Here's how the part is built. I have some questions about the finished solid (model axes, mm). Face numbers are marked on the shaded views. Coordinates: 2 decimals unless noted, no trailing zeros. Write each loop counter-clockwise with the first axis right and the second up, starting at its lowest first coordinate (ties: lowest second). Pieces come first, ordered by that corner, then holes. Notation, with made-up numbers: M 66.5,-37.75 L 85.5,-37.75 A32 ccw 85.5,-4.75 Z; hole C 31,9.5 d6. An arc over 180 degrees is marked long. Use a Markdown table: item, result.
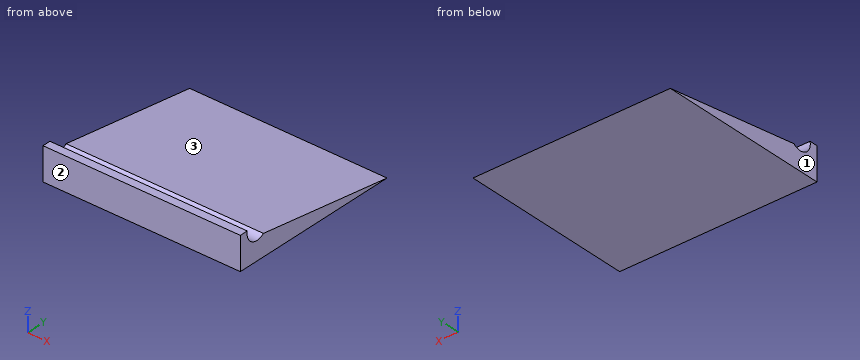
```python
from build123d import *

# Parameters (mm, degrees)
F1_DEPTH = 152.4


with BuildPart() as f1:
    # F0 (on Right) → F1 (new body)
    with BuildSketch(Plane.YZ):
        with BuildLine():
            Line((-92.604421, 0.601124), (-90.45029, 0.601124))
            Line((-90.45029, 0.601124), (41.62971, 0.601124))
            Line((41.62971, 0.601124), (-71.477041, 17.073922))
            ThreePointArc((-71.477041, 17.073922), (-82.034408, 16.292348), (-86.254421, 26.001124))
            Line((-86.254421, 26.001124), (-92.604421, 26.001124))
            Line((-92.604421, 26.001124), (-92.604421, 0.601124))
        make_face()
    extrude(amount=-F1_DEPTH)


solid = f1.part
```
1. Suppose I cut it at B-B on y = -32.5. Write out the boundary of the cut face in (x, z), and give its area (3 significant figures).
Answers follow:
| item | result |
|---|---|
| outline | M -152.4,0.6 L 0,0.6 L 0,11.4 L -152.4,11.4 Z |
| area | 1,650 mm2 |
2. I need wall thicknesses on probe 1 along Z at (x, y) = (-78.5, -67.5); probe 2 along Z at (x, y) = (-65, 28); probe 3 along Y at (x, z) = (-81, 24.75). Which ranges of each line are inside material? Lowest first, please.
Answers follow:
| item | result |
|---|---|
| probe 1 | z = 0.6 to 16.49 |
| probe 2 | z = 0.6 to 2.59 |
| probe 3 | y = -92.6 to -86.43 |
3. Will this pin go through, and if not, where does the flat tip stop? pin 1 Ø1.5 at (x, y) = (-132, -38) entering from +Z.
Answers follow:
| item | result |
|---|---|
| pin 1 | stops at z = 12.31 |
4. Suppose I cut it at C-C on z = 5.75. Write out the boundary of the cut face in (x, y).
Answers follow:
| item | result |
|---|---|
| outline | M -152.4,-92.6 L 0,-92.6 L 0,6.28 L -152.4,6.28 Z |
5. Suppose I cut it at A-A on x = -91.5. Write out the boundary of the cut face in (y, z).
Answers follow:
| item | result |
|---|---|
| outline | M -92.6,0.6 L 41.63,0.6 L -71.48,17.07 A9.14 cw -86.25,26 L -92.6,26 Z |
6. We'd pull the mould along Y, two halves only. Please class the marked faces 1, 2 and 3: +Y half, -Y half, draft (parallel to the pull), parting line (faces both ways), or undercut.
Answers follow:
| item | result |
|---|---|
| face 1 | draft |
| face 2 | -Y half |
| face 3 | +Y half |
